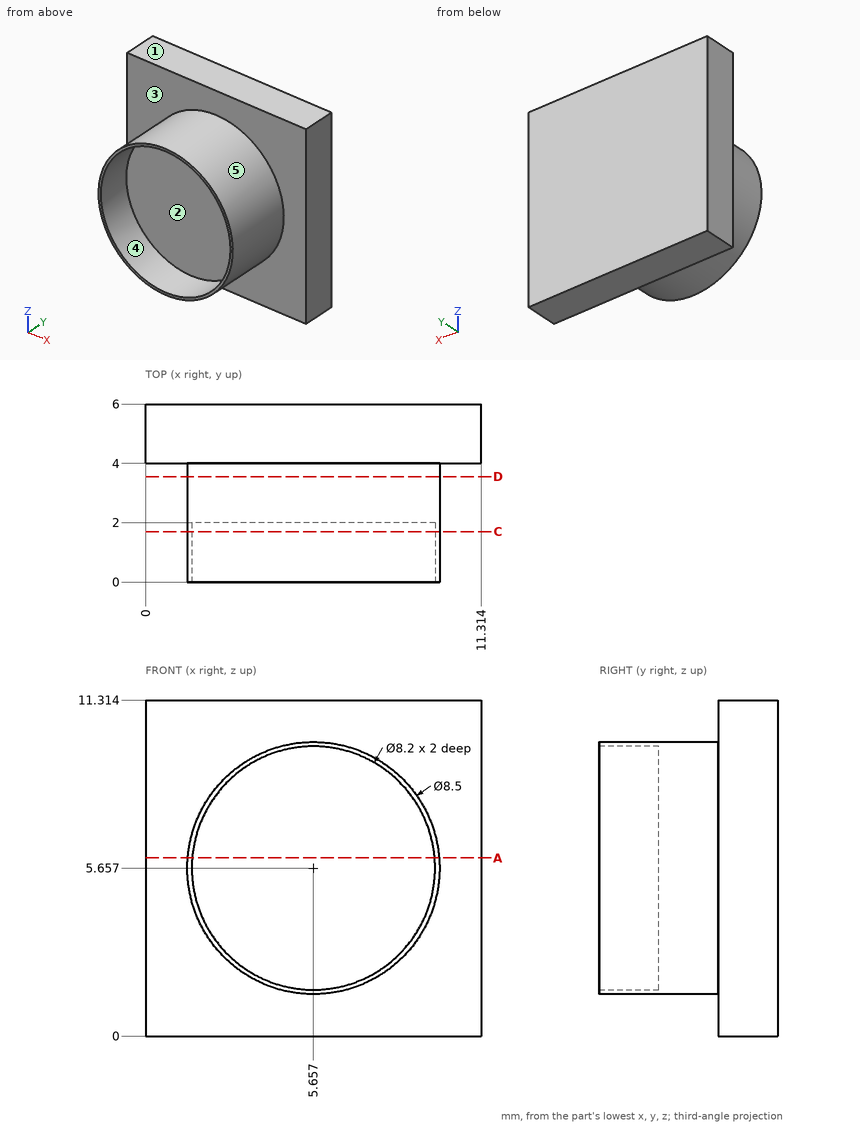
Could you check a few things on this drawing? It's one solid part, dimensions in mm from its lowest x, y, z. A direction names the side the tool comes from. Round coordinates to 2 decimals unless told otherwise and drop trailing zeros. Order: outer loops, then holes, each group sorted by start corner. A loop starts at its lowest first (then second) coordinate and runs counter-clockwise, first axis right, second up. Notation, with made-up numbers: M 82,43.25 L 125,43.25 A14 cw 125,60.25 Z; hole C 25.5,-30.75 d6. An arc over 180 degrees is marked long. One line per question, with ' | ' between items. Start each with the question number.
(1) For P1, Ø6, axis at x = 8.5, z = 7, coming from the -Y side; P2, Ø2.5, axis at x = 6.5, z = 6.5, coming from the -Y side, each with a flat end and sliding along its axis, tell me the tip position at first contact or that it passes through.
(2) Suppose I cut it at D-D on y = 3.55. List the corners of the cut face in (x, z) for me.
(3) Suppose I cut it at C-C on y = 1.7. List the corners of the cut face in (x, z) for me.
(4) Please list where these lines run through material, in increasing order: line 1 along Z through (x, y) = (5.5, 1.45); line 2 along Y through (x, z) = (8, 4.5); line 3 along Z through (x, y) = (5.75, 3.8).
(5) Suppose I cut it at A-A on z = 6. List the corners of the cut face in (x, y) for me.
(6) Thinking about a two-plate mould opening in Z: for the marked faces 3, 4 and 5, which applies, +Z half, -Z half, draft (parallel to the pull), parting line (faces both ways), or undercut?
(7) For the marked faces 1 and 2, which set-ups out of +Z, -Z, +X, -X, +Y, -Y let a thin tool reach every point of the face, with its end or its side?
Geometry results:
1) P1: y = 0 | P2: y = 2
2) outline: C 5.66,5.66 d8.5
3) outline: C 5.66,5.66 d8.5; hole C 5.66,5.66 d8.2
4) line 1: 1.41 to 1.56, 9.75 to 9.9 | line 2: 2 to 6 | line 3: 1.41 to 9.91
5) outline: M 0,4 L 1.42,4 L 1.42,0 L 1.57,0 L 1.57,2 L 9.74,2 L 9.74,0 L 9.89,0 L 9.89,4 L 11.31,4 L 11.31,6 L 0,6 Z
6) face 3: draft | face 4: undercut | face 5: parting line
7) face 1: +Z, +X, -X, +Y, -Y | face 2: -Y
